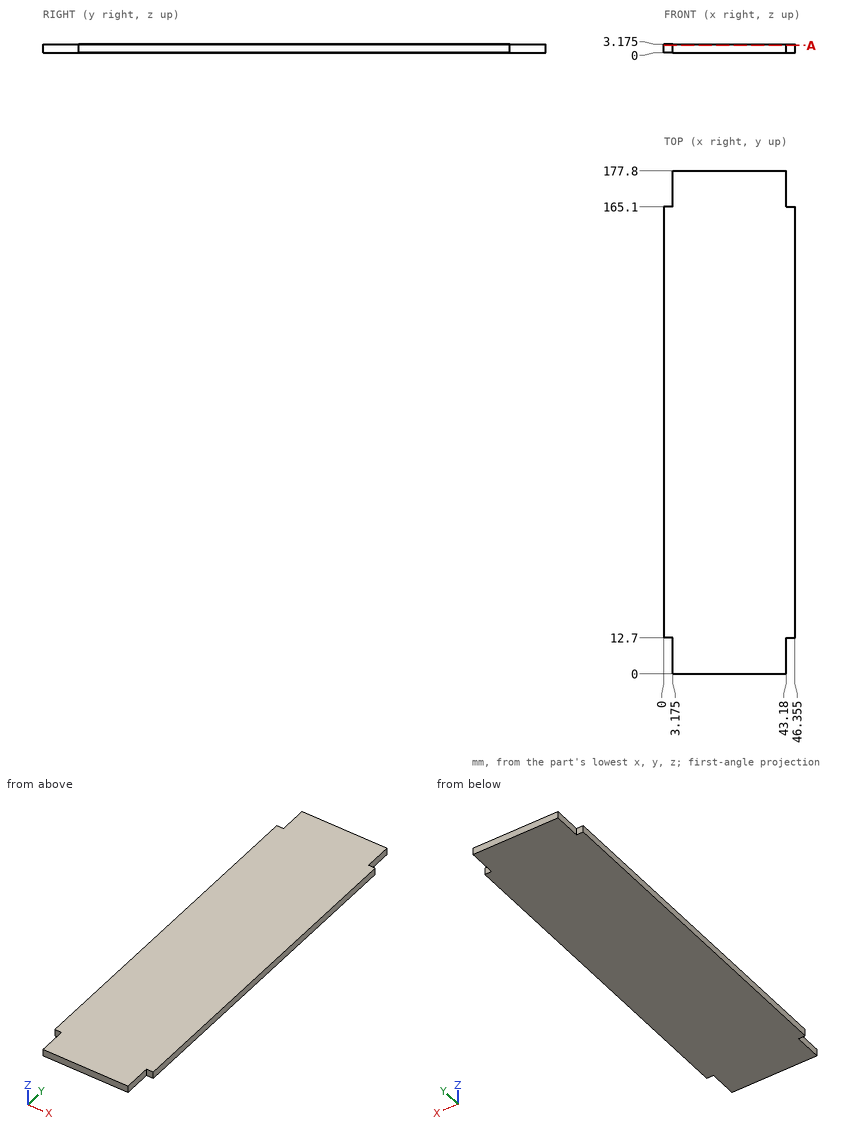
Answer from the drawing. Dimensions are ordinates in mm from the lowest x, y and z of the part. Round coordinates to 2 decimals unless told otherwise and drop trailing zeros. Loops run counter-clockwise (first coordinate to the right, second up) from the corner with the lowest first, then second, coordinate; pieces in that order, holes last. Notation, with made-up numbers: (16.25, -20.75) - (43.25, -20.75) arc R20 cw to (43.25, -8.75) - close; hole circle Ø8 at (-20, -4.5). An arc over 180 degrees is marked (long way). Return JSON: item names as keys, results as strings. Group by question number.
1. Consider probe 1 along X at (y, z) = (11, 2.85) (3 decimals); probe 2 along Y at (x, z) = (43.5, 1.5). Determine where each line is inside the solid, lowest interval first.
2. The part is cut by section A-A on z = 2.65. Determine the outline of the cut face in (x, y) (3 decimals), then the cut area to 3 significant figures.
3. Each of these flat-tipped pins is pushed along its axis until it touches: P1, Ø1, axis at y = 173, z = 1.5, coming from the -X side (3 decimals); P2, Ø1.6, axis at y = 6, z = 1, coming from the +X side; P3, Ø1, axis at x = 44.5, z = 2, coming from the +Y side. Where does it stop, or does it pass through?
Resolved:
{
 "1": {"probe 1": "x = 3.175 to 43.18", "probe 2": "y = 12.7 to 165.1"},
 "2": {"outline": "(0, 12.7) - (3.175, 12.7) - (3.175, 0) - (43.18, 0) - (43.18, 12.7) - (46.355, 12.7) - (46.355, 165.1) - (43.18, 165.1) - (43.18, 177.8) - (3.175, 177.8) - (3.175, 165.1) - (0, 165.1) - close", "area": "8,080 mm²"},
 "3": {"P1": "stops at x = 3.175", "P2": "stops at x = 43.18", "P3": "stops at y = 165.1"}
}
